Here's how the part is built. I have some questions about the finished solid (model axes, mm). Round coordinates to 2 decimals unless told otherwise and drop trailing zeros. Loops run counter-clockwise (first coordinate to the right, second up) from the corner with the lowest first, then second, coordinate; pieces in that order, holes last. Notation, with made-up numbers: (-39, -16) - (-4, -16) arc R18 cw to (-4, -1) - close; hole circle Ø2 at (18.25, 51.25). An arc over 180 degrees is marked (long way). Return JSON: item names as keys, results as strings. Group by question number.
```python
from build123d import *

# Parameters (mm, degrees)
SKETCH_1_R          = 34
SKETCH_1_R_2        = 19
EXTRUDE_1_DEPTH     = 8
SKETCH_2_R          = 2.5
CUT_EXTRUDE_1_DEPTH = 49.744230428


with BuildPart() as part:
    # Эскиз1 → Вытянуть1 (new body)
    with BuildSketch(Plane(origin=(0, 0, 0), x_dir=(1, 0, 0), z_dir=(0, 1, 0))):
        with Locations(Location((0, 0, 0), (0, 0, 270))):
            Circle(SKETCH_1_R)
        with Locations(Location((0, 0, 0), (0, 0, 270))):
            Circle(SKETCH_1_R_2, mode=Mode.SUBTRACT)
    extrude(amount=EXTRUDE_1_DEPTH)

    # Эскиз2 → Вырез-Вытянуть1 (cut, through all)
    with BuildSketch(Plane(origin=(0, 8, 0), x_dir=(1, 0, 0), z_dir=(0, 1, 0))):
        with Locations(Location((0, 29.48960133, 0), (0, 0, 270))):
            Circle(SKETCH_2_R)
        with Locations(Location((29.48960133, 0, 0), (0, 0, 270))):
            Circle(SKETCH_2_R)
        with Locations(Location((0, -29.48960133, 0), (0, 0, 270))):
            Circle(SKETCH_2_R)
        with Locations(Location((-29.48960133, 0, 0), (0, 0, 270))):
            Circle(SKETCH_2_R)
    extrude(amount=-CUT_EXTRUDE_1_DEPTH, mode=Mode.SUBTRACT)


solid = part.part
```
Q1. Please list where these lines run through material, in increasing order: line 1 (X direction, y = 2, z = 0); line 2 (Z direction, x = 29, y = 0.75); line 3 (X direction, y = 2.25, z = 10.5).
Q2. Imagine slicing it at B-B, the plane x = 0. List the corners of the cut face in (y, z) for me, and give its area (3 significant figures).
Q3. Will these pins go through, and if not, where does the flat tip stop? pin 1 Ø2 at (x, y) = (-16, 5.5) entering from +Z; pin 2 Ø4 at (y, z) = (5, -16.5) entering from +X; pin 3 Ø1 at (x, y) = (-25.5, 4.5) entering from -Z.
Q4. Imagine slicing it at A-A, the plane z = 0. List the corners of the cut face in (x, y) for me.
Q5. Imagine slicing it at D-D, the plane x = -28. List the corners of the cut face in (y, z) for me, and give its area (3 significant figures).
Q6. Imagine slicing it at C-C, the plane z = 28. List the corners of the cut face in (x, y) for me, and give its area (3 significant figures).
Q7. If we mould it in two halves opening along X, with no side actions, what happens to faces 1 (the cylindrical face through (27.05, 4.06, -0.54)), 2 (the flat face through (-15, 0, 15)), 3 (the cylindrical face through (33.71, 3.94, -4.43))? For each: +X half, -X half, draft (parallel to the pull), parting line (faces both ways), or undercut.
Output values:
{
 "1": {"line 1": "x = -34 to -31.99, -26.99 to -19, 19 to 26.99, 31.99 to 34", "line 2": "z = -17.75 to -2.45, 2.45 to 17.75", "line 3": "x = -32.34 to -15.84, 15.84 to 32.34"},
 "2": {"outline": "(0, -34) - (8, -34) - (8, -31.99) - (0, -31.99) - close; (0, -26.99) - (8, -26.99) - (8, -19) - (0, -19) - close; (0, 19) - (8, 19) - (8, 26.99) - (0, 26.99) - close; (0, 31.99) - (8, 31.99) - (8, 34) - (0, 34) - close", "area": "160 mm^2"},
 "3": {"pin 1": "stops at z = 30.51", "pin 2": "stops at x = 30.75", "pin 3": "stops at z = -23.04"},
 "4": {"outline": "(-34, 0) - (-31.99, 0) - (-31.99, 8) - (-34, 8) - close; (-26.99, 0) - (-19, 0) - (-19, 8) - (-26.99, 8) - close; (19, 0) - (26.99, 0) - (26.99, 8) - (19, 8) - close; (31.99, 0) - (34, 0) - (34, 8) - (31.99, 8) - close"},
 "5": {"outline": "(0, -19.29) - (8, -19.29) - (8, -2.01) - (0, -2.01) - close; (0, 2.01) - (8, 2.01) - (8, 19.29) - (0, 19.29) - close", "area": "276 mm^2"},
 "6": {"outline": "(-19.29, 0) - (-2.01, 0) - (-2.01, 8) - (-19.29, 8) - close; (2.01, 0) - (19.29, 0) - (19.29, 8) - (2.01, 8) - close", "area": "276 mm^2"},
 "7": {"face 1": "undercut", "face 2": "draft", "face 3": "parting line"}
}
